The drawing under review shows one solid part. Ordinate dimensions are in mm from its lowest x, y, z. Give positions to 0.01 mm unless a question says otherwise; leave off trailing zeros. Write each loop counter-clockwise with the first axis right and the second up, starting at its lowest first coordinate (ties: lowest second). Pieces come first, ordered by that corner, then holes. Notation, with made-up numbers: M 65.25,-38.75 L 109.25,-38.75 A32 ccw 109.25,-0.75 Z; hole C 68.25,34 d1. An arc over 180 degrees is marked long. Answer as a JSON object with one key per item and string values. Group by question number.
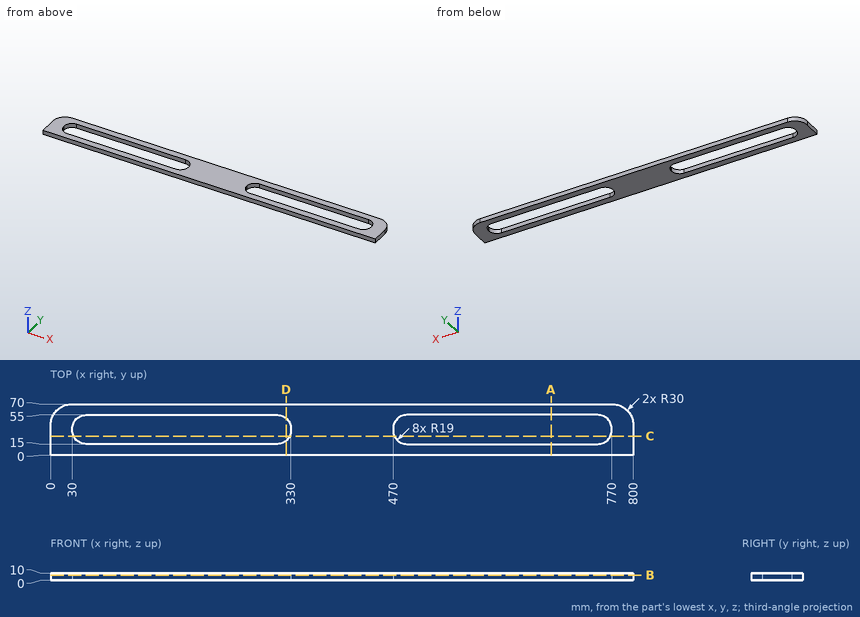
Item 1: Consider section C-C (y = 26). Give the boundary of the cut face in (x, z).
Item 2: Consider section B-B (z = 7.25). Give the boundary of the cut face in (x, y).
Item 3: Consider section D-D (x = 323.5). Give the boundary of the cut face in (y, z), plus the area to 3 significant figures.
Item 4: Insertion check: P1, Ø12, axis at x = 671.5, y = 24.5, coming from the -Z side. The pin has a flat end and moves straight along its axis. Give the tip position at first contact, or say it passes through.
Item 5: Consider section A-A (x = 687). Give the boundary of the cut face in (y, z), plus the area to 3 significant figures.
Item 6: To check wall thickness, follow probe 1 along X at (y, z) = (34, 3.5); probe 2 along X at (y, z) = (52, 3); probe 3 along Y at (x, z) = (282.5, 2.5). State the ranges of each line that lie inside material, in increasing order.
Result set:
{
 "1": {"outline": "M 0,0 L 31.77,0 L 31.77,10 L 0,10 Z; M 328.23,0 L 471.77,0 L 471.77,10 L 328.23,10 Z; M 768.23,0 L 800,0 L 800,10 L 768.23,10 Z"},
 "2": {"outline": "M 0,0 L 800,0 L 800,40 A30 ccw 770,70 L 30,70 A30 ccw 0,40 Z; hole M 30,34 A19 ccw 49,15 L 311,15 A19 ccw 330,34 L 330,36 A19 ccw 311,55 L 49,55 A19 ccw 30,36 Z; hole M 470,34 A19 ccw 489,15 L 751,15 A19 ccw 770,34 L 770,36 A19 ccw 751,55 L 489,55 A19 ccw 470,36 Z"},
 "3": {"outline": "M 0,0 L 19.69,0 L 19.69,10 L 0,10 Z; M 50.31,0 L 70,0 L 70,10 L 50.31,10 Z", "area": "394 mm^2"},
 "4": {"P1": "passes through"},
 "5": {"outline": "M 0,0 L 15,0 L 15,10 L 0,10 Z; M 55,0 L 70,0 L 70,10 L 55,10 Z", "area": "300 mm^2"},
 "6": {"probe 1": "x = 0 to 30, 330 to 470, 770 to 800", "probe 2": "x = 2.5 to 38.75, 321.25 to 478.75, 761.25 to 797.5", "probe 3": "y = 0 to 15, 55 to 70"}
}
